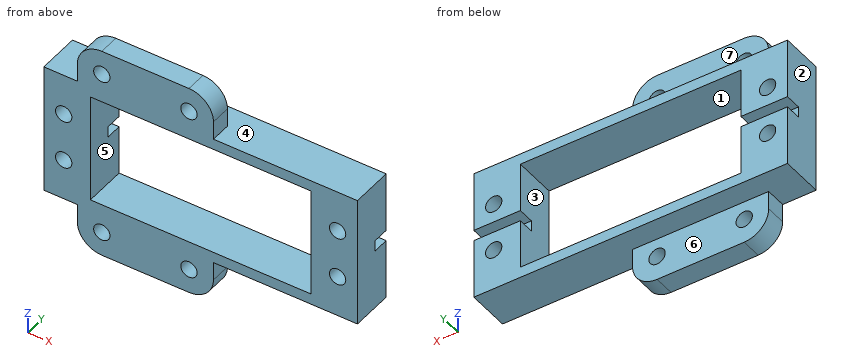
```python
from build123d import *

# Parameters (mm, degrees)
SKETCH1_R             = 1.5
BOSS_EXTRUDE1_DEPTH   = 7.8
BOSS_EXTRUDE1_2_DEPTH = 7.8
SKETCH2_W             = 2
SKETCH2_H             = 20
BOSS_EXTRUDE2_DEPTH   = 7.8
SKETCH3_W             = 8.55
SKETCH3_H             = 0.1
BOSS_EXTRUDE3_DEPTH   = 7.8
SKETCH4_W             = 57.6
SKETCH4_H             = 2
BOSS_EXTRUDE4_DEPTH   = 7.8
SKETCH5_W             = 8.55
SKETCH5_H             = 2
CUT_EXTRUDE1_DEPTH    = 3
SKETCH6_R             = 1.5
BOSS_EXTRUDE5_DEPTH   = 7.8
SKETCH7_R             = 1.5
CUT_EXTRUDE2_DEPTH    = 4


with BuildPart() as part:
    # Sketch1 → Boss-Extrude1 (new body)
    with BuildSketch(Plane(origin=(0, 0, 0), x_dir=(1, 0, 0), z_dir=(0, 1, 0))):
        Polygon((-54.762761852, 25.466548835), (-54.762761852, 5.466548835), (-48.212761852, 5.466548835), (-48.212761852, 12.451776091), (-48.212761852, 18.48132158), (-48.212761852, 25.466548835), align=None)
        with Locations(Location((-49.862761852, 10.966548835, 0), (0, 0, 270))):
            Circle(SKETCH1_R, mode=Mode.SUBTRACT)
        with Locations(Location((-49.862761852, 19.966548835, 0), (0, 0, 270))):
            Circle(SKETCH1_R, mode=Mode.SUBTRACT)
    extrude(amount=BOSS_EXTRUDE1_DEPTH)



with BuildPart() as body_2:
    # Sketch1 → Boss-Extrude1 2 (new body)
    with BuildSketch(Plane(origin=(0, 0, 0), x_dir=(1, 0, 0), z_dir=(0, 1, 0))):
        Polygon((-101.812761852, 18.48132158), (-101.812761852, 12.451776091), (-101.812761852, 5.466548835), (-101.212761852, 5.466548835), (-95.262761852, 5.466548835), (-95.262761852, 25.466548835), (-101.812761852, 25.466548835), (-101.812761852, 24.866548835), (-101.812761852, 21.451776091), align=None)
        with Locations(Location((-100.162761852, 10.966548835, 0), (0, 0, 270))):
            Circle(SKETCH1_R, mode=Mode.SUBTRACT)
        with Locations(Location((-100.162761852, 19.966548835, 0), (0, 0, 270))):
            Circle(SKETCH1_R, mode=Mode.SUBTRACT)
    extrude(amount=BOSS_EXTRUDE1_2_DEPTH)


with BuildPart() as part_1:
    add(part.part)

    add(body_2.part)  # Boss-Extrude2 merges body 2
    # Sketch2 → Boss-Extrude2 (add)
    with BuildSketch(Plane(origin=(0, 7.8, 0), x_dir=(1, 0, 0), z_dir=(0, 1, 0))):
        with Locations((-47.212761852, 15.466548835)):
            Rectangle(SKETCH2_W, SKETCH2_H)
        with Locations((-102.812761852, 15.466548835)):
            Rectangle(SKETCH2_W, SKETCH2_H)
    extrude(amount=-BOSS_EXTRUDE2_DEPTH)

    # Sketch3 → Boss-Extrude3 (add)
    with BuildSketch(Plane(origin=(0, 7.8, 0), x_dir=(1, 0, 0), z_dir=(0, 1, 0))):
        with Locations((-99.537761852, 5.416548835)):
            Rectangle(SKETCH3_W, SKETCH3_H)
        with Locations((-99.537761852, 25.516548835)):
            Rectangle(SKETCH3_W, SKETCH3_H)
        with Locations((-50.487761852, 25.516548835)):
            Rectangle(SKETCH3_W, SKETCH3_H)
        with Locations((-50.487761852, 5.416548835)):
            Rectangle(SKETCH3_W, SKETCH3_H)
    extrude(amount=-BOSS_EXTRUDE3_DEPTH)

    # Sketch4 → Boss-Extrude4 (add)
    with BuildSketch(Plane(origin=(0, 7.8, 0), x_dir=(1, 0, 0), z_dir=(0, 1, 0))):
        with Locations((-75.012761852, 26.566548835)):
            Rectangle(SKETCH4_W, SKETCH4_H)
        with Locations((-75.012761852, 4.366548835)):
            Rectangle(SKETCH4_W, SKETCH4_H)
    extrude(amount=-BOSS_EXTRUDE4_DEPTH)

    # Sketch5 → Cut-Extrude1 (cut)
    with BuildSketch(Plane(origin=(0, 7.8, 0), x_dir=(1, 0, 0), z_dir=(0, 1, 0))):
        with Locations((-99.537761852, 15.466548835)):
            Rectangle(SKETCH5_W, SKETCH5_H)
        with Locations((-50.487761852, 15.466548835)):
            Rectangle(SKETCH5_W, SKETCH5_H)
    extrude(amount=-CUT_EXTRUDE1_DEPTH, mode=Mode.SUBTRACT)

    # Sketch6 → Boss-Extrude5 (add)
    # profile 1 of 10: a face of its own
    with BuildSketch(Plane(origin=(0, 7.8, 0), x_dir=(1, 0, 0), z_dir=(0, 1, 0))):
        with BuildLine():
            Line((-97.660965944, 3.366548835), (-97.660965944, -0.033392238))
            ThreePointArc((-97.660965944, -0.033392238), (-97.254605431, 1.835328112), (-96.108914501, 3.366548835))
            Line((-96.108914501, 3.366548835), (-97.660965944, 3.366548835))
        make_face()
    # profile 2 of 10: a face of its own
    with BuildSketch(Plane(origin=(0, 7.8, 0), x_dir=(1, 0, 0), z_dir=(0, 1, 0))):
        with BuildLine():
            ThreePointArc((-96.108914501, 3.366548835), (-97.254605431, 1.835328112), (-97.660965944, -0.033392238))
            ThreePointArc((-97.660965944, -0.033392238), (-96.342946459, -3.215372753), (-93.160965944, -4.533392238))
            ThreePointArc((-93.160965944, -4.533392238), (-89.978985428, -3.215372753), (-88.660965944, -0.033392238))
            ThreePointArc((-88.660965944, -0.033392238), (-89.067326456, 1.835328112), (-90.213017386, 3.366548835))
            Line((-90.213017386, 3.366548835), (-96.108914501, 3.366548835))
        make_face()
        with Locations(Location((-93.160965944, -0.033392238, 0), (0, 0, 270))):
            Circle(SKETCH6_R, mode=Mode.SUBTRACT)
    # profile 3 of 10: a face of its own
    with BuildSketch(Plane(origin=(0, 7.8, 0), x_dir=(1, 0, 0), z_dir=(0, 1, 0))):
        with BuildLine():
            ThreePointArc((-88.660965944, -0.033392238), (-89.978985428, -3.215372753), (-93.160965944, -4.533392238))
            Line((-93.160965944, -4.533392238), (-77.160965417, -4.533392238))
            ThreePointArc((-77.160965417, -4.533392238), (-81.376990489, -1.606647648), (-80.108913974, 3.366548835))
            Line((-80.108913974, 3.366548835), (-90.213017386, 3.366548835))
            ThreePointArc((-90.213017386, 3.366548835), (-89.067326456, 1.835328112), (-88.660965944, -0.033392238))
        make_face()
    # profile 4 of 10: a face of its own
    with BuildSketch(Plane(origin=(0, 7.8, 0), x_dir=(1, 0, 0), z_dir=(0, 1, 0))):
        with BuildLine():
            ThreePointArc((-80.108913974, 3.366548835), (-81.376990489, -1.606647648), (-77.160965417, -4.533392238))
            ThreePointArc((-77.160965417, -4.533392238), (-73.978984901, -3.215372753), (-72.660965417, -0.033392238))
            ThreePointArc((-72.660965417, -0.033392238), (-73.067325929, 1.835328112), (-74.213016859, 3.366548835))
            Line((-74.213016859, 3.366548835), (-80.108913974, 3.366548835))
        make_face()
        with Locations(Location((-77.160965417, -0.033392238, 0), (0, 0, 270))):
            Circle(SKETCH6_R, mode=Mode.SUBTRACT)
    # profile 5 of 10: a face of its own
    with BuildSketch(Plane(origin=(0, 7.8, 0), x_dir=(1, 0, 0), z_dir=(0, 1, 0))):
        with BuildLine():
            ThreePointArc((-74.213016859, 3.366548835), (-73.067325929, 1.835328112), (-72.660965417, -0.033392238))
            Line((-72.660965417, -0.033392238), (-72.660965417, 3.366548835))
            Line((-72.660965417, 3.366548835), (-74.213016859, 3.366548835))
        make_face()
    # profile 6 of 10: a face of its own
    with BuildSketch(Plane(origin=(0, 7.8, 0), x_dir=(1, 0, 0), z_dir=(0, 1, 0))):
        with BuildLine():
            ThreePointArc((-72.660965417, 30.966605859), (-73.978984901, 34.148586374), (-77.160965417, 35.466605859))
            ThreePointArc((-77.160965417, 35.466605859), (-81.377021429, 32.539778353), (-80.108780241, 27.566548835))
            Line((-80.108780241, 27.566548835), (-74.213150592, 27.566548835))
            ThreePointArc((-74.213150592, 27.566548835), (-73.067362681, 29.097805001), (-72.660965417, 30.966605859))
        make_face()
        with Locations(Location((-77.160965417, 30.966605859, 0), (0, 0, 270))):
            Circle(SKETCH6_R, mode=Mode.SUBTRACT)
    # profile 7 of 10: a face of its own
    with BuildSketch(Plane(origin=(0, 7.8, 0), x_dir=(1, 0, 0), z_dir=(0, 1, 0))):
        with BuildLine():
            Line((-74.213150592, 27.566548835), (-72.660965417, 27.566548835))
            Line((-72.660965417, 27.566548835), (-72.660965417, 30.966605859))
            ThreePointArc((-72.660965417, 30.966605859), (-73.067362681, 29.097805001), (-74.213150592, 27.566548835))
        make_face()
    # profile 8 of 10: a face of its own
    with BuildSketch(Plane(origin=(0, 7.8, 0), x_dir=(1, 0, 0), z_dir=(0, 1, 0))):
        with BuildLine():
            Line((-77.160965417, 35.466605859), (-93.160965944, 35.466605859))
            ThreePointArc((-93.160965944, 35.466605859), (-89.978985428, 34.148586374), (-88.660965944, 30.966605859))
            ThreePointArc((-88.660965944, 30.966605859), (-89.067363208, 29.097805001), (-90.213151119, 27.566548835))
            Line((-90.213151119, 27.566548835), (-80.108780241, 27.566548835))
            ThreePointArc((-80.108780241, 27.566548835), (-81.377021429, 32.539778353), (-77.160965417, 35.466605859))
        make_face()
    # profile 9 of 10: a face of its own
    with BuildSketch(Plane(origin=(0, 7.8, 0), x_dir=(1, 0, 0), z_dir=(0, 1, 0))):
        with BuildLine():
            ThreePointArc((-93.160965944, 35.466605859), (-96.342946459, 34.148586374), (-97.660965944, 30.966605859))
            ThreePointArc((-97.660965944, 30.966605859), (-97.254568679, 29.097805001), (-96.108780768, 27.566548835))
            Line((-96.108780768, 27.566548835), (-90.213151119, 27.566548835))
            ThreePointArc((-90.213151119, 27.566548835), (-89.067363208, 29.097805001), (-88.660965944, 30.966605859))
            ThreePointArc((-88.660965944, 30.966605859), (-89.978985428, 34.148586374), (-93.160965944, 35.466605859))
        make_face()
        with Locations(Location((-93.160965944, 30.966605859, 0), (0, 0, 270))):
            Circle(SKETCH6_R, mode=Mode.SUBTRACT)
    # profile 10 of 10: a face of its own
    with BuildSketch(Plane(origin=(0, 7.8, 0), x_dir=(1, 0, 0), z_dir=(0, 1, 0))):
        with BuildLine():
            Line((-97.660965944, 30.966605859), (-97.660965944, 27.566548835))
            Line((-97.660965944, 27.566548835), (-96.108780768, 27.566548835))
            ThreePointArc((-96.108780768, 27.566548835), (-97.254568679, 29.097805001), (-97.660965944, 30.966605859))
        make_face()
    extrude(amount=-BOSS_EXTRUDE5_DEPTH)

    # Sketch7 → Cut-Extrude2 (cut)
    # profile 1 of 2: a face of its own
    with BuildSketch(Plane(origin=(0, 7.8, 0), x_dir=(1, 0, 0), z_dir=(0, 1, 0))):
        with BuildLine():
            Line((-97.660965944, 3.366548835), (-72.660965417, 3.366548835))
            Line((-72.660965417, 3.366548835), (-72.660965417, -0.033392238))
            ThreePointArc((-72.660965417, -0.033392238), (-73.978984901, -3.215372753), (-77.160965417, -4.533392238))
            Line((-77.160965417, -4.533392238), (-93.160965944, -4.533392238))
            ThreePointArc((-93.160965944, -4.533392238), (-96.342946459, -3.215372753), (-97.660965944, -0.033392238))
            Line((-97.660965944, -0.033392238), (-97.660965944, 3.366548835))
        make_face()
        with Locations(Location((-77.160965417, -0.033392238, 0), (0, 0, 270))):
            Circle(SKETCH7_R, mode=Mode.SUBTRACT)
        with Locations(Location((-93.160965944, -0.033392238, 0), (0, 0, 270))):
            Circle(SKETCH7_R, mode=Mode.SUBTRACT)
    # profile 2 of 2: a face of its own
    with BuildSketch(Plane(origin=(0, 7.8, 0), x_dir=(1, 0, 0), z_dir=(0, 1, 0))):
        with BuildLine():
            Line((-77.160965417, 35.466605859), (-93.160965944, 35.466605859))
            ThreePointArc((-93.160965944, 35.466605859), (-96.342946459, 34.148586374), (-97.660965944, 30.966605859))
            Line((-97.660965944, 30.966605859), (-97.660965944, 27.566548835))
            Line((-97.660965944, 27.566548835), (-72.660965417, 27.566548835))
            Line((-72.660965417, 27.566548835), (-72.660965417, 30.966605859))
            ThreePointArc((-72.660965417, 30.966605859), (-73.978984901, 34.148586374), (-77.160965417, 35.466605859))
        make_face()
    extrude(amount=-CUT_EXTRUDE2_DEPTH, mode=Mode.SUBTRACT)


solid = part_1.part
```
Build history of the part. All positions in model axes, mm. Face numbers are marked on the shaded views. A direction names the side the tool comes from. Coordinates: 2 decimals unless noted, no trailing zeros. Order: outer loops, then holes, each group sorted by start corner. A loop starts at its lowest first (then second) coordinate and runs counter-clockwise, first axis right, second up.
Item 1: Drill centre lines: L1, parallel to X at y = 3, z = -7; L2, parallel to Z at x = -76, y = 0.5; L3, parallel to Z at x = -83, y = 4. Where is each one in solid material? Low to high.
Filled in:
L1: x = -103.81 to -95.26, -54.76 to -46.21
L2: z = -35.31 to -31.92, -30.02 to -25.57, -5.37 to -0.92, 0.98 to 4.38
L3: z = -27.57 to -25.57, -5.37 to -3.37
Item 2: Saw through at A-A on x = -66.5. List the corners of the cut face in (y, z), then the cut area to 3 significant figures.
Filled in:
outline: (0, -27.57) - (7.8, -27.57) - (7.8, -25.57) - (0, -25.57) - close; (0, -5.37) - (7.8, -5.37) - (7.8, -3.37) - (0, -3.37) - close
area: 31.2 mm2
Item 3: Mould opens along X. For the marked faces 1, 2, 3 and 4 say: released by +X, released by -X, zero draft, split by the parting line, or undercut.
Filled in:
face 1: undercut
face 2: released by -X
face 3: undercut
face 4: zero draft
Item 4: Saw through at C-C on y = 6. List the corners of the cut face in (x, z).
Filled in:
outline: (-103.81, -27.57) - (-46.21, -27.57) - (-46.21, -16.47) - (-54.76, -16.47) - (-54.76, -25.57) - (-95.26, -25.57) - (-95.26, -16.47) - (-103.81, -16.47) - close; (-103.81, -14.47) - (-95.26, -14.47) - (-95.26, -5.37) - (-54.76, -5.37) - (-54.76, -14.47) - (-46.21, -14.47) - (-46.21, -3.37) - (-103.81, -3.37) - close; hole circle Ø3 at (-100.16, -19.97); hole circle Ø3 at (-100.16, -10.97); hole circle Ø3 at (-49.86, -19.97); hole circle Ø3 at (-49.86, -10.97)
Item 5: Saw through at D-D on y = 2.75. State how many separate pieces and enclosed holes the cut face has, then the cut area to 3 significant figures.
Filled in:
separate pieces: 1
enclosed holes: 9
area: 897 mm2
Item 6: Drop flat-ended pins along their axis: pin 1 Ø4 at (x, y) = (-74.5, 2) entering from +Z; pin 2 Ø2.5 at (x, y) = (-49.5, 5.5) entering from -Z; pin 3 Ø2 at (x, y) = (-75.5, 2) entering from -Z. Give the stop position or say it passes through.
Filled in:
pin 1: stops at z = 4.48
pin 2: stops at z = -27.57
pin 3: stops at z = -35.42
Item 7: Tool access for the marked faces 5, 6 and 7: list every direction of +Z, -Z, +X, -X, +Y, -Y with a clear straight run to the whole face (end or side of a thin tool).
Filled in:
face 5: +Y, -Y
face 6: -Z, +X, -X, +Y
face 7: +Z, +X, -X, +Y
Item 8: Saw through at B-B on z = -25. List the corners of the cut face in (x, y), then the cut area to 3 significant figures.
Filled in:
outline: (-103.81, 0) - (-95.26, 0) - (-95.26, 7.8) - (-103.81, 7.8) - close; (-54.76, 0) - (-46.21, 0) - (-46.21, 7.8) - (-54.76, 7.8) - close
area: 133 mm2
